Check sheet for the modelled part. Datum: model origin and axes. Units: mm. A direction names the side the tool comes from. Round coordinates to 2 decimals unless told otherwise and drop trailing zeros. Write each loop counter-clockwise with the first axis right and the second up, starting at its lowest first coordinate (ties: lowest second). Pieces come first, ordered by that corner, then holes.
Item 1: Cross-section at A-A on x = -31.75. Enter the section's corners in (y, z) (3 decimals), plus the area to 3 significant figures.
Item 2: Go/stop test with flat-tipped pins: pin 1 Ø4 at (x, z) = (29, -11.5) entering from +Y; pin 2 Ø5 at (x, z) = (-31.75, 12.7) entering from +Y. Record where each tip stops, or that it passes through.
Item 3: Cross-section at C-C on y = 7.5. Enter the section's corners in (x, z).
Item 4: Tool access check on faces 4 (the flat face through (-1, 0, -29)), 5 (the flat face through (-34.5, 6.35, 15.4)). Record the directions out of +Z, -Z, +X, -X, +Y, -Y that give a thin tool (end or side, any length) a straight path to the whole face; none if there is none.
Item 5: Material ranges on line 1 (Z direction, x = -31.75, y = 3.75) (3 decimals); line 2 (X direction, y = 4.5, z = 0); line 3 (X direction, y = 9.75, z = 12.7), recorded low to high.
Item 6: Cross-section at D-D on x = 0. Enter the section's corners in (y, z).
Item 7: Release check for a two-part mould opening along Z. For faces 1 (the cylindrical face through (33.657, 9.569, -6.643)), 2 (the flat face through (-1, 12.7, 28)), 3 (the flat face through (-1, 6, 31.75)) record: +Z half, -Z half, draft (parallel to the pull), parting line (faces both ways), or undercut.
Item 8: Cross-section at B-B on z = 0. Enter the section's corners in (x, y), plus the area to 3 significant figures.
from build123d import *

# Parameters (mm, degrees)
SKETCH1_W           = 88.9
SKETCH1_H           = 63.5
SKETCH1_R           = 25.654
SKETCH1_R_2         = 3.175
BOSS_EXTRUDE1_DEPTH = 12.7
FILLET1_R           = 5.08
SKETCH2_R           = 6.35
CUT_EXTRUDE1_DEPTH  = 6.35


with BuildPart() as part:
    # Sketch1 → Boss-Extrude1 (new body)
    with BuildSketch(Plane(origin=(0, 0, 0), x_dir=(1, 0, 0), z_dir=(0, 1, 0))):
        Rectangle(SKETCH1_W, SKETCH1_H)
        with Locations(Location((0, 0, 0), (0, 0, 270))):
            Circle(SKETCH1_R, mode=Mode.SUBTRACT)
        with Locations(Location((-31.75, 12.7, 0), (0, 0, 270))):
            Circle(SKETCH1_R_2, mode=Mode.SUBTRACT)
        with Locations(Location((-31.75, -12.7, 0), (0, 0, 270))):
            Circle(SKETCH1_R_2, mode=Mode.SUBTRACT)
        with Locations(Location((31.75, -12.7, 0), (0, 0, 270))):
            Circle(SKETCH1_R_2, mode=Mode.SUBTRACT)
        with Locations(Location((31.75, 12.7, 0), (0, 0, 270))):
            Circle(SKETCH1_R_2, mode=Mode.SUBTRACT)
    extrude(amount=BOSS_EXTRUDE1_DEPTH)

    # Fillet1
    fillet1_edges = [part.edges().sort_by_distance(p)[0] for p in [
        (44.45, 6.35, 31.75),
        (-44.45, 6.35, 31.75),
        (-44.45, 6.35, -31.75),
        (44.45, 6.35, -31.75),
    ]]
    fillet(fillet1_edges, radius=FILLET1_R)

    # Sketch2 → Cut-Extrude1 (cut)
    with BuildSketch(Plane(origin=(0, 12.7, 0), x_dir=(1, 0, 0), z_dir=(0, 1, 0))):
        with Locations(Location((-31.75, 12.7, 0), (0, 0, 270))):
            Circle(SKETCH2_R)
        with Locations(Location((-31.75, -12.7, 0), (0, 0, 270))):
            Circle(SKETCH2_R)
        with Locations(Location((31.75, -12.7, 0), (0, 0, 270))):
            Circle(SKETCH2_R)
        with Locations(Location((31.75, 12.7, 0), (0, 0, 270))):
            Circle(SKETCH2_R)
    extrude(amount=-CUT_EXTRUDE1_DEPTH, mode=Mode.SUBTRACT)


solid = part.part
Response values:
1. outline: (0, -31.75) - (12.7, -31.75) - (12.7, -19.05) - (6.35, -19.05) - (6.35, -15.875) - (0, -15.875) - close; (0, -9.525) - (6.35, -9.525) - (6.35, -6.35) - (12.7, -6.35) - (12.7, 6.35) - (6.35, 6.35) - (6.35, 9.525) - (0, 9.525) - close; (0, 15.875) - (6.35, 15.875) - (6.35, 19.05) - (12.7, 19.05) - (12.7, 31.75) - (0, 31.75) - close
1. area: 565 mm2
2. pin 1: stops at y = 6.35
2. pin 2: passes through
3. outline: (-44.45, -26.67) arc R5.08 ccw to (-39.37, -31.75) - (39.37, -31.75) arc R5.08 ccw to (44.45, -26.67) - (44.45, 26.67) arc R5.08 ccw to (39.37, 31.75) - (-39.37, 31.75) arc R5.08 ccw to (-44.45, 26.67) - close; hole circle Ø12.7 at (-31.75, -12.7); hole circle Ø12.7 at (-31.75, 12.7); hole circle Ø51.31 at (0, 0); hole circle Ø12.7 at (31.75, -12.7); hole circle Ø12.7 at (31.75, 12.7)
4. face 4: +Z, -Z, +X, -X, -Y
4. face 5: +Y
5. line 1: z = -31.75 to -15.875, -9.525 to 9.525, 15.875 to 31.75
5. line 2: x = -44.45 to -25.65, 25.65 to 44.45
5. line 3: x = -44.45 to -38.1, -25.4 to -22.29, 22.29 to 25.4, 38.1 to 44.45
6. outline: (0, -31.75) - (12.7, -31.75) - (12.7, -25.65) - (0, -25.65) - close; (0, 25.65) - (12.7, 25.65) - (12.7, 31.75) - (0, 31.75) - close
7. face 1: undercut
7. face 2: draft
7. face 3: +Z half
8. outline: (-44.45, 0) - (-25.65, 0) - (-25.65, 12.7) - (-44.45, 12.7) - close; (25.65, 0) - (44.45, 0) - (44.45, 12.7) - (25.65, 12.7) - close
8. area: 477 mm2
